```python
from build123d import *

# Parameters (mm, degrees)
SKETCH_1_W          = 103
SKETCH_1_H          = 103
EXTRUDE_1_DEPTH     = 1.5
SKETCH_3_W          = 103
SKETCH_3_H          = 103
SKETCH_3_W_2        = 100
SKETCH_3_H_2        = 100
EXTRUDE_2_DEPTH     = 8.5
SKETCH_4_R          = 1
CUT_EXTRUDE_1_DEPTH = 1.5


with BuildPart() as part:
    # 草图1 → 凸台-拉伸1 (new body)
    with BuildSketch(Plane.XY):
        with Locations((51.5, -51.5)):
            Rectangle(SKETCH_1_W, SKETCH_1_H)
    extrude(amount=EXTRUDE_1_DEPTH)

    # 草图3 → 凸台-拉伸2 (add)
    with BuildSketch(Plane.XY.offset(1.5)):
        with Locations((51.5, -51.5)):
            Rectangle(SKETCH_3_W, SKETCH_3_H)
        with Locations((51.5, -51.5)):
            Rectangle(SKETCH_3_W_2, SKETCH_3_H_2, mode=Mode.SUBTRACT)
    extrude(amount=EXTRUDE_2_DEPTH)

    # 草图4 → 切除-拉伸1 (cut)
    with BuildSketch(Plane.XY.offset(1.5)):
        with Locations((4.126355777, -98.5)):
            Circle(SKETCH_4_R)
        with Locations((98.5, -98.5)):
            Circle(SKETCH_4_R)
        with Locations((98.5, -4.5)):
            Circle(SKETCH_4_R)
        with Locations((4.5, -4.5)):
            Circle(SKETCH_4_R)
    extrude(amount=-CUT_EXTRUDE_1_DEPTH, mode=Mode.SUBTRACT)


solid = part.part
```
Design review of the part built by this model. Coordinates are the model's own, in mm. A direction names the side the tool comes from. Give positions to 0.01 mm unless a question says otherwise; leave off trailing zeros. Write each loop counter-clockwise with the first axis right and the second up, starting at its lowest first coordinate (ties: lowest second). Pieces come first, ordered by that corner, then holes. Notation, with made-up numbers: (-10.75, 10.25) -> (43.25, 10.25) arc R18 cw to (43.25, 33.25) -> close; hole circle Ø1 at (58.5, 21). An arc over 180 degrees is marked (long way). Answer in a Markdown table with one row per item.
(1) To check wall thickness, follow probe 1 along X at (y, z) = (-98.5, 0.55); probe 2 along Y at (x, z) = (98.5, 0.4); probe 3 along X at (y, z) = (-71, 7.5). State the ranges of each line that lie inside material, in increasing order.
Results:
| item | result |
|---|---|
| probe 1 | 0 to 3.13, 5.13 to 97.5, 99.5 to 103 |
| probe 2 | -103 to -99.5, -97.5 to -5.5, -3.5 to 0 |
| probe 3 | 0 to 1.5, 101.5 to 103 |
(2) Consider section A-A (z = 3.75). State the section outline as (x, y) points, then the cut area to 3 significant figures.
Results:
| item | result |
|---|---|
| outline | (0, -103) -> (103, -103) -> (103, 0) -> (0, 0) -> close; hole (1.5, -101.5) -> (101.5, -101.5) -> (101.5, -1.5) -> (1.5, -1.5) -> close |
| area | 609 mm2 |
(3) Clearance check with a flat-ended pin moving along its axis: pin 1 (2.5 mm diameter, centred on x = 4.5, y = -4.5, fed in from +Z). State where the tip first meets the part, or that it passes through.
Results:
| item | result |
|---|---|
| pin 1 | z = 1.5 |
(4) Consider section B-B (y = -45). State the section outline as (x, z) points, then the cut area to 3 significant figures.
Results:
| item | result |
|---|---|
| outline | (0, 0) -> (103, 0) -> (103, 10) -> (101.5, 10) -> (101.5, 1.5) -> (1.5, 1.5) -> (1.5, 10) -> (0, 10) -> close |
| area | 180 mm2 |
(5) Consider section C-C (x = 94). State the section outline as (y, z) points, then the cut area to 3 significant figures.
Results:
| item | result |
|---|---|
| outline | (-103, 0) -> (0, 0) -> (0, 10) -> (-1.5, 10) -> (-1.5, 1.5) -> (-101.5, 1.5) -> (-101.5, 10) -> (-103, 10) -> close |
| area | 180 mm2 |
(6) For faces 1 (the flat face through (51, 0, 5)), 2 (the flat face through (51, -51, 1.5)), list the 3-axis set-ups (+Z, -Z, +X, -X, +Y, -Y) from which the entire face can be reached by the end or side of a thin tool; tool diameter is ignored.
Results:
| item | result |
|---|---|
| face 1 | +Z, -Z, +X, -X, +Y |
| face 2 | +Z |
(7) Mouldability with a two-part tool opening along X and no side actions: class faces 3 (the flat face through (0, -52, 5)), 4 (the flat face through (103, -52, 5)), 5 (the flat face through (101.5, -52, 6)), 6 (the flat face through (51, -51, 0)) as +X half, -X half, draft (parallel to the pull), parting line (faces both ways), or undercut.
Results:
| item | result |
|---|---|
| face 3 | -X half |
| face 4 | +X half |
| face 5 | undercut |
| face 6 | draft |
